```python
from build123d import *

# Parameters (mm, degrees)
BOSS_EXTRUDE3_DEPTH = 28
FILLET1_R           = 10
SKETCH8_R           = 9.5
SKETCH8_W           = 8
SKETCH8_H           = 5
CUT_EXTRUDE4_DEPTH  = 5
SKETCH9_R           = 1.75
CUT_EXTRUDE5_DEPTH  = 20
SKETCH10_R          = 1.75
CUT_EXTRUDE6_DEPTH  = 10
CUT_EXTRUDE8_DEPTH  = 10
CHAMFER1_SIZE       = 6.5
FILLET3_R           = 4
CUT_EXTRUDE9_DEPTH  = 5


# Some blends are built 0.0001 mm under size
with BuildPart() as part:
    # Sketch7 → Boss-Extrude3 (new body)
    with BuildSketch(Plane.XY):
        with BuildLine():
            Line((-29.009414831, -4.685297633), (114.990585169, -4.685297633))
            ThreePointArc((114.990585169, -4.685297633), (122.279275038, -2.340345638), (126.833304451, 3.814702367))
            Line((126.833304451, 3.814702367), (134.833304451, 3.814702367))
            Line((134.833304451, 3.814702367), (134.833304451, 7.314702367))
            Line((134.833304451, 7.314702367), (127.480581166, 7.314702367))
            Line((127.480581166, 7.314702367), (124.47741815, 7.314702367))
            ThreePointArc((124.47741815, 7.314702367), (105.490585169, 7.814702367), (124.47741815, 8.314702367))
            Line((124.47741815, 8.314702367), (127.480581166, 8.314702367))
            Line((127.480581166, 8.314702367), (134.833304451, 8.314702367))
            Line((134.833304451, 8.314702367), (134.833304451, 11.814702367))
            Line((134.833304451, 11.814702367), (126.833304451, 11.814702367))
            ThreePointArc((126.833304451, 11.814702367), (125.854338173, 13.997652364), (124.47741815, 15.954112665))
            Line((124.47741815, 15.954112665), (124.47741815, 32.314702367))
            Line((124.47741815, 32.314702367), (96.47741815, 32.314702367))
            Line((96.47741815, 32.314702367), (96.47741815, 0.314702367))
            Line((96.47741815, 0.314702367), (-10.496247811, 0.314702367))
            Line((-10.496247811, 0.314702367), (-10.496247811, 32.314702367))
            Line((-10.496247811, 32.314702367), (-38.496247811, 32.314702367))
            Line((-38.496247811, 32.314702367), (-38.496247811, 15.954112665))
            ThreePointArc((-38.496247811, 15.954112665), (-39.873167835, 13.997652364), (-40.852134113, 11.814702367))
            Line((-40.852134113, 11.814702367), (-48.852134113, 11.814702367))
            Line((-48.852134113, 11.814702367), (-48.852134113, 8.314702367))
            Line((-48.852134113, 8.314702367), (-41.499410828, 8.314702367))
            Line((-41.499410828, 8.314702367), (-38.496247811, 8.314702367))
            ThreePointArc((-38.496247811, 8.314702367), (-19.509414831, 7.814702367), (-38.496247811, 7.314702367))
            Line((-38.496247811, 7.314702367), (-41.499410828, 7.314702367))
            Line((-41.499410828, 7.314702367), (-48.852134113, 7.314702367))
            Line((-48.852134113, 7.314702367), (-48.852134113, 3.814702367))
            Line((-48.852134113, 3.814702367), (-40.852134113, 3.814702367))
            ThreePointArc((-40.852134113, 3.814702367), (-36.298104699, -2.340345638), (-29.009414831, -4.685297633))
        make_face()
    extrude(amount=BOSS_EXTRUDE3_DEPTH)

    # Fillet1
    fillet1_edges = [part.edges().sort_by_distance(p)[0] for p in [
        (-10.496247811, 0.314702367, 14),
        (96.47741815, 0.314702367, 14),
    ]]
    fillet(fillet1_edges, radius=FILLET1_R)

    # Sketch8 → Cut-Extrude4 (cut)
    with BuildSketch(Plane(origin=(0, 0.314702367, 0), x_dir=(1, 0, 0), z_dir=(0, 1, 0))):
        with Locations(Location((63.990585169, -14, 0), (0, 0, 270))):
            Circle(SKETCH8_R)
        with Locations(Location((21.990585169, -14, 0), (0, 0, 270))):
            Circle(SKETCH8_R)
        with Locations((42.990585169, -14)):
            Rectangle(SKETCH8_W, SKETCH8_H)
    extrude(amount=-CUT_EXTRUDE4_DEPTH, mode=Mode.SUBTRACT)

    # Sketch9 → Cut-Extrude5 (cut)
    with BuildSketch(Plane(origin=(0, 11.814702367, 0), x_dir=(1, 0, 0), z_dir=(0, 1, 0))):
        with Locations(Location((130.833304451, -14, 0), (0, 0, 270))):
            Circle(SKETCH9_R)
        with Locations(Location((-44.852134113, -14, 0), (0, 0, 180))):
            Circle(SKETCH9_R)
    extrude(amount=-CUT_EXTRUDE5_DEPTH, mode=Mode.SUBTRACT)

    # Sketch10 → Cut-Extrude6 (cut)
    with BuildSketch(Plane(origin=(0, 32.314702367, 0), x_dir=(1, 0, 0), z_dir=(0, 1, 0))):
        with Locations(Location((110.490585169, -14, 0), (0, 0, 180))):
            Circle(SKETCH10_R)
        with Locations(Location((-24.509414831, -14, 0), (0, 0, 180))):
            Circle(SKETCH10_R)
    extrude(amount=-CUT_EXTRUDE6_DEPTH, mode=Mode.SUBTRACT)

    # Sketch12 → Cut-Extrude8 (cut)
    with BuildSketch(Plane(origin=(0, 11.814702367, 0), x_dir=(1, 0, 0), z_dir=(0, 1, 0))):
        Polygon((130.833304451, -21.5), (126.833304451, -21.5), (126.833304451, -28), (134.833304451, -28), (134.833304451, -21.5), align=None)
        Polygon((130.833304451, -6.5), (126.833304451, -6.5), (126.833304451, 0), (134.833304451, 0), (134.833304451, -6.5), align=None)
        Polygon((-44.852134113, -6.5), (-40.852134113, -6.5), (-40.852134113, 0), (-48.852134113, 0), (-48.852134113, -6.5), align=None)
        Polygon((-44.852134113, -21.5), (-48.852134113, -21.5), (-48.852134113, -28), (-40.852134113, -28), (-40.852134113, -21.5), align=None)
    extrude(amount=-CUT_EXTRUDE8_DEPTH, mode=Mode.SUBTRACT)

    # Chamfer1
    chamfer1_edges = [part.edges().sort_by_distance(p)[0] for p in [
        (126.833304451, 10.064702367, 6.5),
        (126.833304451, 5.564702367, 6.5),
        (126.833304451, 5.564702367, 21.5),
        (126.833304451, 10.064702367, 21.5),
        (-40.852134113, 5.564702367, 21.5),
        (-40.852134113, 5.564702367, 6.5),
        (-40.852134113, 10.064702367, 6.5),
        (-40.852134113, 10.064702367, 21.5),
    ]]
    chamfer(chamfer1_edges, length=CHAMFER1_SIZE - 0.0001)  # a hair under: the kernel refuses the full size

    # Fillet3
    # the kernel refuses this fillet: 4 mm, written as the material it takes off along each edge
    with BuildSketch(Plane(origin=(134.833304451, 19.621150019, 21.5), x_dir=(-1, 0, 0), z_dir=(0, -1, 0))) as fillet3_piece_1:
        with BuildLine():
            CenterArc((4, 3.122579061), FILLET3_R, 180, 51.319647456)
            Line((0, 3.122579061), (-0.08, 3.122579061))
            Line((-0.08, 3.122579061), (-0.08, 0))
            Line((-0.08, 0), (0, -0.08))
            ThreePointArc((0, -0.08), (0.75005, -0.08), (1.450102, -0.062451581))
            Line((1.450102, -0.062451581), (1.5001, 0))
        make_face()
    extrude(amount=19.112895303, mode=Mode.SUBTRACT)
    with BuildSketch(Plane(origin=(134.833304451, 15.121150019, 21.5), x_dir=(0, 0, -1), z_dir=(0, -1, 0)), Plane(origin=(-48.852134113, 15.121150019, 6.5), x_dir=(0, 0, 1), z_dir=(0, -1, 0)), Plane(origin=(-48.852134113, 19.621150019, 6.5), x_dir=(0, 0, 1), z_dir=(0, -1, 0))) as fillet3_piece_2:
        with BuildLine():
            CenterArc((3.122579061, -4), FILLET3_R, 90, 51.319647456)
            Line((0, -1.5001), (-0.062451581, -1.450102))
            ThreePointArc((-0.062451581, -1.450102), (-0.08, -0.75005), (-0.08, 0))
            Line((-0.08, 0), (0, 0.08))
            Line((0, 0.08), (3.122579061, 0.08))
            Line((3.122579061, 0.08), (3.122579061, 0))
        make_face()
    extrude(amount=19.112895303, mode=Mode.SUBTRACT)
    with BuildSketch(Plane(origin=(134.833304451, 15.121150019, 6.5), x_dir=(0, 0, 1), z_dir=(0, -1, 0)), Plane(origin=(134.833304451, 19.621150019, 6.5), x_dir=(0, 0, 1), z_dir=(0, -1, 0)), Plane(origin=(-48.852134113, 19.621150019, 21.5), x_dir=(0, 0, -1), z_dir=(0, -1, 0))) as fillet3_piece_3:
        with BuildLine():
            CenterArc((3.122579061, 4), FILLET3_R, 218.680352544, 51.319647456)
            Line((0, 1.5001), (-0.062451581, 1.450102))
            ThreePointArc((-0.062451581, 1.450102), (-0.08, 0.75005), (-0.08, 0))
            Line((-0.08, 0), (0, -0.08))
            Line((0, -0.08), (3.122579061, -0.08))
            Line((3.122579061, -0.08), (3.122579061, 0))
        make_face()
    extrude(amount=19.112895303, mode=Mode.SUBTRACT)
    with BuildSketch(Plane(origin=(-48.852134113, 15.121150019, 21.5), x_dir=(1, 0, 0), z_dir=(0, -1, 0))) as fillet3_piece_4:
        with BuildLine():
            CenterArc((4, -3.122579061), FILLET3_R, 128.680352544, 51.319647456)
            Line((0, -3.122579061), (-0.08, -3.122579061))
            Line((-0.08, -3.122579061), (-0.08, 0))
            Line((-0.08, 0), (0, 0.08))
            ThreePointArc((0, 0.08), (0.75005, 0.08), (1.450102, 0.062451581))
            Line((1.450102, 0.062451581), (1.5001, 0))
        make_face()
    extrude(amount=19.112895303, mode=Mode.SUBTRACT)

    # Sketch13 → Cut-Extrude9 (cut)
    with BuildSketch(Plane(origin=(0, 32.314702367, 0), x_dir=(1, 0, 0), z_dir=(0, 1, 0))):
        Polygon((108.614196794, -17.25), (112.366973544, -17.25), (114.243361919, -14), (112.366973544, -10.75), (108.614196794, -10.75), (106.737808419, -14), align=None)
        Polygon((-20.756638081, -14), (-22.633026456, -10.75), (-26.385803206, -10.75), (-28.262191581, -14), (-26.385803206, -17.25), (-22.633026456, -17.25), align=None)
    extrude(amount=-CUT_EXTRUDE9_DEPTH, mode=Mode.SUBTRACT)


solid = part.part
```
Here's how the part is built. I have some questions about the finished solid (model axes, mm). A direction names the side the tool comes from. Round coordinates to 2 decimals unless told otherwise and drop trailing zeros. Order: outer loops, then holes, each group sorted by start corner. A loop starts at its lowest first (then second) coordinate and runs counter-clockwise, first axis right, second up. Notation, with made-up numbers: M 7,42.5 L 25,42.5 A19 cw 25,66.5 Z; hole C 7.25,6 d2. An arc over 180 degrees is marked long. Answer in a Markdown table with one row per item.
Item 1: Imagine slicing it at D-D, the plane x = 60. Write out the boundary of the cut face in (y, z).
A:
| item | result |
|---|---|
| outline | M -4.69,0 L 0.31,0 L 0.31,5.38 L -4.69,5.38 Z; M -4.69,22.62 L 0.31,22.62 L 0.31,28 L -4.69,28 Z |
Item 2: Imagine slicing it at C-C, the plane x = 9. Write out the boundary of the cut face in (y, z).
A:
| item | result |
|---|---|
| outline | M -4.69,0 L 0.31,0 L 0.31,28 L -4.69,28 Z |
Item 3: If I drill on L1, parallel to Z at x = 42, y = -2; L2, parallel to X at y = 19, z = 6.5; L3, parallel to X at y = 9.5, z = 3, over which ranges is the centre line in solid material (lowest first)? Write a range as from..to.
A:
| item | result |
|---|---|
| L1 | z = 0..11.5, 16.5..28 |
| L2 | x = -38.5..-10.5, 96.48..124.48 |
| L3 | x = -43.85..-38.36, -19.66..-10.46, 96.44..105.64, 124.34..129.83 |
Item 4: I'm going to push flat-ended pins straight in: pin 1 (5 mm diameter, centred on x = 127.5, z = 11.5, fed in from +Y); pin 2 (4 mm diameter, centred on x = 130, z = 20.5, fed in from +Y); pin 3 (3 mm diameter, centred on x = -25, z = 13.5, fed in from +Y). Where does each tip first touch, or does it pass through?
A:
| item | result |
|---|---|
| pin 1 | stops at y = 15.3 |
| pin 2 | stops at y = 11.81 |
| pin 3 | stops at y = 27.31 |
Item 5: Imagine slicing it at B-B, the plane z = 26. Write out the boundary of the cut face in (x, y).
A:
| item | result |
|---|---|
| outline | M -42.85,3.81 L -40.85,3.81 A12.5 ccw -29.01,-4.69 L 114.99,-4.69 A12.5 ccw 126.83,3.81 L 128.83,3.81 L 128.83,7.31 L 124.48,7.31 A9.5 cw long 124.48,8.31 L 128.83,8.31 L 128.83,11.81 L 126.83,11.81 A12.5 ccw 124.48,15.95 L 124.48,32.31 L 96.48,32.31 L 96.48,10.31 A10 cw 86.48,0.31 L -0.5,0.31 A10 cw -10.5,10.31 L -10.5,32.31 L -38.5,32.31 L -38.5,15.95 A12.5 ccw -40.85,11.81 L -42.85,11.81 L -42.85,8.31 L -38.5,8.31 A9.5 cw long -38.5,7.31 L -42.85,7.31 Z |
Item 6: Thinking about a two-plate mould opening in X: for faces 1 (the face through (-44.15, 10.09, 3.3)), 2 (the face through (42, -4.685, 11)), 3 (the face through (-22.9, 27.315, 15.4)), which applies, +X half, -X half, draft (parallel to the pull), parting line (faces both ways), or undercut?
A:
| item | result |
|---|---|
| face 1 | -X half |
| face 2 | draft |
| face 3 | undercut |
Item 7: Imagine slicing it at A-A, the plane x = -31.5. Write out the boundary of the cut face in (y, z).
A:
| item | result |
|---|---|
| outline | M -4.43,0 L -1.35,0 L -1.35,28 L -4.43,28 Z; M 16.98,0 L 32.31,0 L 32.31,28 L 16.98,28 Z |
Item 8: For faces 4 (the face through (128, 3.815, 14)), 5 (the face through (38.991, -2, 14)), 6 (the face through (-25.45, 24.85, 15.476)), 7 (the face through (128.6, 7.315, 13.8)), 8 (the face through (-42.6, 8.315, 13.8)), which set-ups out of +Z, -Z, +X, -X, +Y, -Y let a thin tool reach every point of the face, with its end or its side?
A:
| item | result |
|---|---|
| face 4 | +Z, -Z, +X, -Y |
| face 5 | +Y, -Y |
| face 6 | +Y |
| face 7 | +Z, -Z, +X |
| face 8 | +Z, -Z, -X |
